```python
from build123d import *

# Parameters (mm, degrees)
SKETCH1_W           = 10
SKETCH1_H           = 70
BOSS_EXTRUDE1_DEPTH = 1.5
SKETCH2_W           = 2
SKETCH2_H           = 1.5
CUT_EXTRUDE1_DEPTH  = 10
SKETCH3_W           = 0.2
SKETCH3_H           = 60
CUT_EXTRUDE2_DEPTH  = 10


with BuildPart() as part:
    # Sketch1 → Boss-Extrude1 (new body)
    with BuildSketch(Plane(origin=(0, 0, 0), x_dir=(0, 0, -1), z_dir=(1, 0, 0))):
        with Locations((-5, 4.155844156)):
            Rectangle(SKETCH1_W, SKETCH1_H)
    extrude(amount=BOSS_EXTRUDE1_DEPTH)

    # Sketch2 → Cut-Extrude1 (cut)
    with BuildSketch(Plane(origin=(1.5, 0, 0), x_dir=(0, 0, -1), z_dir=(1, 0, 0))):
        with Locations((-9, 38.405844156)):
            Rectangle(SKETCH2_W, SKETCH2_H)
        with Locations((-1, 38.405844156)):
            Rectangle(SKETCH2_W, SKETCH2_H)
        with Locations((-1, -30.094155844)):
            Rectangle(SKETCH2_W, SKETCH2_H)
        with Locations((-9, -30.094155844)):
            Rectangle(SKETCH2_W, SKETCH2_H)
    extrude(amount=-CUT_EXTRUDE1_DEPTH, mode=Mode.SUBTRACT)

    # Sketch3 → Cut-Extrude2 (cut)
    with BuildSketch(Plane(origin=(1.5, 0, 0), x_dir=(0, 0, -1), z_dir=(1, 0, 0))):
        with Locations((-5, 4.155844156)):
            Rectangle(SKETCH3_W, SKETCH3_H)
    extrude(amount=-CUT_EXTRUDE2_DEPTH, mode=Mode.SUBTRACT)


solid = part.part
```
Could you check a few things on this model? Use its own coordinates, in mm. A direction names the side the tool comes from. Round coordinates to 2 decimals unless told otherwise and drop trailing zeros. Write each loop counter-clockwise with the first axis right and the second up, starting at its lowest first coordinate (ties: lowest second). Pieces come first, ordered by that corner, then holes. Notation, with made-up numbers: M 20.5,14 L 66.5,14 A12 ccw 66.5,23 Z; hole C 83.25,43 d5. An arc over 180 degrees is marked long. Write each question's results on one line, items separated by ' | '. Start each with the question number.
1. Imagine slicing it at B-B on x = 0.25. List the corners of the cut face in (y, z) for me, and give its area (3 significant figures).
2. Thinking about a two-plate mould opening in Z: for faces 1 (the face through (1, 4, 5.1)), 2 (the face through (1, 38, 2)), 3 (the face through (1, -30.844, 5)), which applies, +Z half, -Z half, draft (parallel to the pull), parting line (faces both ways), or undercut?
3. Imagine slicing it at A-A on y = 5.5. List the corners of the cut face in (x, z) for me.
4. I need wall thicknesses on L1, parallel to Z at x = 0.25, y = -16; L2, parallel to Y at x = 0.2, z = 5; L3, parallel to Y at x = 0.9, z = 8.5. Which ranges of each line are inside material? Lowest first, please. Write a range as from..to.
5. On a 3-axis mill with a long thin cutter (end or side, diameter ignored), from which of +Z, -Z, +X, -X, +Y, -Y can I reach the whole of each face in a straight line? I mean faces 4 (the face through (1, 37.656, 1)), 5 (the face through (1, -30, 8)), 6 (the face through (1, -30, 2)), 7 (the face through (1, 38, 8)). Say none if no direction works.
Result sheet:
1) outline: M -30.84,2 L -29.34,2 L -29.34,0 L 37.66,0 L 37.66,2 L 39.16,2 L 39.16,8 L 37.66,8 L 37.66,10 L -29.34,10 L -29.34,8 L -30.84,8 Z; hole M -25.84,4.9 L 34.16,4.9 L 34.16,5.1 L -25.84,5.1 Z | area: 676 mm^2
2) face 1: undercut | face 2: -Z half | face 3: draft
3) outline: M 0,0 L 1.5,0 L 1.5,4.9 L 0,4.9 Z; M 0,5.1 L 1.5,5.1 L 1.5,10 L 0,10 Z
4) L1: z = 0..4.9, 5.1..10 | L2: y = -30.84..-25.84, 34.16..39.16 | L3: y = -29.34..37.66
5) face 4: -Z, +X, -X, +Y | face 5: +Z, +X, -X, -Y | face 6: -Z, +X, -X, -Y | face 7: +Z, +X, -X, +Y
